Geometry: final body of the model. Coordinates: model frame, mm. A direction names the side the tool comes from. Give positions to 0.01 mm unless a question says otherwise; leave off trailing zeros. Order: outer loops, then holes, each group sorted by start corner. A loop starts at its lowest first (then second) coordinate and runs counter-clockwise, first axis right, second up. Notation, with made-up numbers: (65, -22.75) - (77, -22.75) arc R27 ccw to (77, -5.75) - close; hole circle Ø4 at (73, -35.5). An arc over 180 degrees is marked (long way). One line per item, written item: value.
```python
from build123d import *

# Parameters (mm, degrees)
SKETCH1_R               = 28.4
SKETCH1_R_2             = 3
SKETCH1_R_3             = 2.6
BOSS_EXTRUDE1_DEPTH     = 6
SKETCH3_R               = 12
BOSS_EXTRUDE2_DEPTH     = 24
SKETCH1_3_R             = 3
CUT_EXTRUDE1_DEPTH      = 24
CUT_EXTRUDE2_REACH      = 48.788
CUT_EXTRUDE2_END_RADIUS = 12
SKETCH4_R               = 2.5


with BuildPart() as part:
    # Sketch1 → Boss-Extrude1 (new body)
    # profile 1 of 2: a face of its own
    with BuildSketch(Plane.XY):
        Circle(SKETCH1_R)
        Circle(SKETCH1_R_2, mode=Mode.SUBTRACT)
        with Locations((-20.56810334, 11.875)):
            Circle(SKETCH1_R_3, mode=Mode.SUBTRACT)
        with Locations((-20.56810334, -11.875)):
            Circle(SKETCH1_R_3, mode=Mode.SUBTRACT)
        with Locations((0, -23.75)):
            Circle(SKETCH1_R_3, mode=Mode.SUBTRACT)
        with Locations((20.56810334, -11.875)):
            Circle(SKETCH1_R_3, mode=Mode.SUBTRACT)
        with Locations((20.56810334, 11.875)):
            Circle(SKETCH1_R_3, mode=Mode.SUBTRACT)
        with Locations((0, 23.75)):
            Circle(SKETCH1_R_3, mode=Mode.SUBTRACT)
    # profile 2 of 2: a face of its own
    with BuildSketch(Plane.XY):
        Circle(SKETCH1_R_2)
    extrude(amount=BOSS_EXTRUDE1_DEPTH)

    # Sketch3 → Boss-Extrude2 (add)
    with BuildSketch(Plane(origin=(0, 0, 0), x_dir=(-1, 0, 0), z_dir=(0, 0, -1))):
        Circle(SKETCH3_R)
    extrude(amount=-BOSS_EXTRUDE2_DEPTH)

    # Sketch1<3> → Cut-Extrude1 (cut)
    with BuildSketch(Plane.XY):
        with Locations(Location((0, 0, 0), (0, 0, 180))):
            Circle(SKETCH1_3_R)
    extrude(amount=CUT_EXTRUDE1_DEPTH, mode=Mode.SUBTRACT)

    # Cut-Extrude2: up to this cylinder (the profile starts inside it)
    cut_extrude2_end = Plane(origin=(0, 0, 13.8), z_dir=(0, 0, -1)) * Cylinder(CUT_EXTRUDE2_END_RADIUS, 122.576, mode=Mode.PRIVATE)
    # Sketch4 → Cut-Extrude2 (cut, up to the surface)
    with BuildSketch(Plane(origin=(0, 0, 0), x_dir=(1, 0, 0), z_dir=(0, 1, 0)), mode=Mode.PRIVATE) as cut_extrude2_sk1:
        with Locations(Location((0, -13.8, 0), (0, 0, 90))):
            Circle(SKETCH4_R)
    cut_extrude2_tool1 = extrude(cut_extrude2_sk1.sketch, amount=CUT_EXTRUDE2_REACH, mode=Mode.PRIVATE) & cut_extrude2_end
    add(cut_extrude2_tool1.solids().sort_by_distance((0, 0, 13.8))[0], mode=Mode.SUBTRACT)


solid = part.part
```
1) Section C-C, the plane y = 25. Return loops of the section in (x, z), then the cut area to 3 significant figures.
Answers below:
outline: (-13.47, 0) - (-2.28, 0) - (-2.28, 6) - (-13.47, 6) - close; (2.28, 0) - (13.47, 0) - (13.47, 6) - (2.28, 6) - close
area: 134 mm^2
2) Section D-D, the plane z = 22. Return loops of the section in (x, y).
Answers below:
outline: circle Ø24 at (0, 0); hole circle Ø6 at (0, 0)
3) Mould query, pull axis X, two halves, no side actions, for faces 4 (the face through (21.77, 9.57, 2.96)), 5 (the face through (-3.697, 28.158, 2.958)), 6 (the face through (0, -3, 12)), 7 (the face through (-6, 0, 0)). Classes: released by +X, released by -X, zero draft, split by the parting line, or undercut.
Answers below:
face 4: undercut
face 5: split by the parting line
face 6: undercut
face 7: zero draft
4) First-contact query: pin 1 (4.5 mm diameter, centred on x = 0, z = 13.8, fed in from +Y); pin 2 (5 mm diameter, centred on y = -4, z = 3.5, fed in from -X); pin 3 (6 mm diameter, centred on y = -11, z = 17.5, fed in from -X). Flat tips, straight axial feed; report the tip coordinate or a pass-through.
Answers below:
pin 1: y = -1.98
pin 2: x = -28.36
pin 3: x = -8.94
5) Set-up query: faces 1 (the face through (12.2, 0.4, 6)), 2 (the face through (-0.751, 6.76, 11.415)), 3 (the face through (-2.5, -2.5, 24)). Return all of +Z, -Z, +X, -X, +Y, -Y with unobstructed straight access to the full face (end or side cutting, diameter ignored); none if empty.
Answers below:
face 1: +Z
face 2: +Y
face 3: +Z, +X, -X, +Y, -Y
6) Material intervals for line 1 along Y through (x, z) = (0, 6.5); line 2 along Y through (x, z) = (18.5, 2); line 3 along Z through (x, y) = (21.5, 14.5), sorted ascending.
Answers below:
line 1: -12 to -3, 3 to 12
line 2: -21.55 to -13.45, -10.3 to 10.3, 13.45 to 21.55
line 3: 0 to 6
7) Section B-B, the plane y = -10. Return loops of the section in (x, z), then the cut area to 3 significant figures.
Answers below:
outline: (-26.58, 0) - (-22.37, 0) - (-22.37, 6) - (-26.58, 6) - close; (-18.77, 0) - (18.77, 0) - (18.77, 6) - (6.63, 6) - (6.63, 24) - (-6.63, 24) - (-6.63, 6) - (-18.77, 6) - close; (22.37, 0) - (26.58, 0) - (26.58, 6) - (22.37, 6) - close
area: 515 mm^2
8) Section A-A, the plane x = 0. Return loops of the section in (y, z).
Answers below:
outline: (-28.4, 0) - (-26.35, 0) - (-26.35, 6) - (-28.4, 6) - close; (-21.15, 0) - (-3, 0) - (-3, 24) - (-12, 24) - (-12, 6) - (-21.15, 6) - close; (3, 0) - (21.15, 0) - (21.15, 6) - (12, 6) - (12, 11.3) - (3, 11.3) - close; (3, 16.3) - (12, 16.3) - (12, 24) - (3, 24) - close; (26.35, 0) - (28.4, 0) - (28.4, 6) - (26.35, 6) - close
